```python
from build123d import *

# Parameters (mm, degrees)
F0_R     = 15
F0_R_2   = 3.65
F1_DEPTH = 8
F2_R     = 15
F3_DEPTH = 4
F4_SIZE  = 5
F5_R     = 4.75
F6_DEPTH = 2.5
F7_R     = 2.25
F8_DEPTH = 5
F9_DEPTH = 12


with BuildPart() as f1:
    # F0 (on Top) → F1 (new body)
    with BuildSketch(Plane.XY):
        Circle(F0_R)
        Circle(F0_R_2, mode=Mode.SUBTRACT)
    extrude(amount=F1_DEPTH)

    # F2 (on face) → F3 (join)
    with BuildSketch(Plane.XY.offset(8)):
        Circle(F2_R)
    extrude(amount=F3_DEPTH)

    # F4
    f4_edges = [f1.edges().sort_by_distance(p)[0] for p in [
        (-15, 0, 12),
    ]]
    chamfer(f4_edges, length=F4_SIZE)

    # F5 (on face) → F6 (join)
    with BuildSketch(Plane.XY.offset(12)):
        Circle(F5_R)
    extrude(amount=F6_DEPTH)

    # F7 (on face) → F8 (cut)
    with BuildSketch(Plane.XY.offset(14.5)):
        Circle(F7_R)
    extrude(amount=-F8_DEPTH, mode=Mode.SUBTRACT)

    # F0 (on Top) → F9 (cut)
    with BuildSketch(Plane.XY):
        Circle(F0_R_2)
    extrude(amount=F9_DEPTH, mode=Mode.SUBTRACT)


solid = f1.part
```
Geometry: final body of the model. Coordinates: model frame, mm. A direction names the side the tool comes from. Give positions to 0.01 mm unless a question says otherwise; leave off trailing zeros. Write each loop counter-clockwise with the first axis right and the second up, starting at its lowest first coordinate (ties: lowest second). Pieces come first, ordered by that corner, then holes.
1. Pin query (flat end, axial travel): P1, Ø1.5, axis at x = 5.5, z = 2, coming from the -Y side; P2, Ø3, axis at x = 5.5, y = -5, coming from the +Z side; P3, Ø6, axis at y = 5, z = 4, coming from the -X side. Return the tip coordinate at first contact, or that it passes through.
2. Line query: probe 1 along Y at (x, z) = (0, 6.25); probe 2 along Y at (x, z) = (0, 13.05); probe 3 along X at (y, z) = (-1.75, 6.25). Output: solid intervals per line, ascending.
3. Reachability of faces 1 (the flat face through (-2, -2, 12)), 2 (the cylindrical face through (-0.29, 2.23, 13.27)), 3 (the flat face through (4.3, 2.4, 12)) from +Z, -Z, +X, -X, +Y, -Y: full face, straight path, thin tool, end or side. Return the list, or none.
4. Section query A-A, the plane y = 0. Return loops of the section in (x, z), then the cut area to 3 significant figures.
5. Section query D-D, the plane z = 8.75. Return loops of the section in (x, y), then the cut area to 3 significant figures.
6. Section query C-C, the plane z = 12.75. Return loops of the section in (x, y), then the cut area to 3 significant figures.
7. Draft query along X for faces 4 (the flat face through (3, -3, 0)), 5 (the conical face through (9.77, 3.077, 11.757)), 6 (the cylindrical face through (3.48, 1.1, 5.92)). Return one class per face: released by +X, released by -X, zero draft, split by the parting line, or undercut.
Computed:
1. P1: stops at y = -14.23
1. P2: stops at z = 12
1. P3: stops at x = -14.87
2. probe 1: y = -15 to -3.65, 3.65 to 15
2. probe 2: y = -4.75 to -2.25, 2.25 to 4.75
2. probe 3: x = -14.9 to -3.2, 3.2 to 14.9
3. face 1: -Z
3. face 2: +Z, -Z
3. face 3: +Z
4. outline: (-15, 0) - (-3.65, 0) - (-3.65, 12) - (-2.25, 12) - (-2.25, 14.5) - (-4.75, 14.5) - (-4.75, 12) - (-10, 12) - (-15, 7) - close; (2.25, 12) - (3.65, 12) - (3.65, 0) - (15, 0) - (15, 7) - (10, 12) - (4.75, 12) - (4.75, 14.5) - (2.25, 14.5) - close
4. area: 260 mm2
5. outline: circle Ø26.5 at (0, 0); hole circle Ø7.3 at (0, 0)
5. area: 510 mm2
6. outline: circle Ø9.5 at (0, 0); hole circle Ø4.5 at (0, 0)
6. area: 55.0 mm2
7. face 4: zero draft
7. face 5: split by the parting line
7. face 6: undercut
